```python
from build123d import *

# Parameters (mm, degrees)
SKETCH_1_R          = 1.45
EXTRUDE_1_DEPTH     = 21
EXTRUDE_2_DEPTH     = 1.3
FILLET_1_R          = 0.3
FILLET_2_R          = 0.3
SKETCH_3_R          = 1
CUT_EXTRUDE_3_DEPTH = 10
FILLET_3_R          = 2
SKETCH_4_W          = 3.3
SKETCH_4_H          = 21
EXTRUDE_4_DEPTH     = 0.6
SKETCH_7_W          = 15
SKETCH_7_H          = 13.536537926
SKETCH_7_W_2        = 10.5
SKETCH_7_H_2        = 9.5
CUT_EXTRUDE_4_DEPTH = 10
FILLET_7_R          = 3


with BuildPart() as part:
    # 草圖1 → 填料-伸長1 (new body)
    with BuildSketch(Plane(origin=(0, 0, 0), x_dir=(1, 0, 0), z_dir=(0, 1, 0))):
        Polygon((17.3, -0.9), (14.5, -0.9), (14.5, -4.2), (17.3, -4.2), (17.3, -5), (0, -5), (-2.5, -5), (-2.5, 0), (0, 0), (17.3, 0), align=None)
        with Locations(Location((0, -2.5, 0), (0, 0, 90))):
            Circle(SKETCH_1_R, mode=Mode.SUBTRACT)
    extrude(amount=EXTRUDE_1_DEPTH)

    # 草圖2 → 填料-伸長2 (add)
    with BuildSketch(Plane(origin=(14.5, 0, 0), x_dir=(0, 0, -1), z_dir=(1, 0, 0))):
        Polygon((-4.2, 5.659075235), (-0.9, 4.159075235), (-0.9, 3.5), (-4.2, 5), align=None)
        Polygon((-4.2, 2.659075235), (-0.9, 1.159075235), (-0.9, 0.5), (-4.2, 2), align=None)
        Polygon((-4.2, 17.659075235), (-0.9, 16.159075235), (-0.9, 15.5), (-4.2, 17), align=None)
        Polygon((-4.2, 20.659075235), (-0.9, 19.159075235), (-0.9, 18.5), (-4.2, 20), align=None)
    extrude(amount=EXTRUDE_2_DEPTH)

    # 圓角1
    fillet_1_edges = [part.edges().sort_by_distance(p)[0] for p in [
        (15.8, 1.909075235, 2.55),
        (15.8, 1.25, 2.55),
        (15.8, 4.25, 2.55),
        (15.8, 4.909075235, 2.55),
        (15.8, 16.25, 2.55),
        (15.8, 16.909075235, 2.55),
        (15.8, 19.25, 2.55),
        (15.8, 19.909075235, 2.55),
    ]]
    fillet(fillet_1_edges, radius=FILLET_1_R - 0.0001)  # a hair under: the kernel refuses the full size

    # 圓角2
    fillet_2_edges = [part.edges().sort_by_distance(p)[0] for p in [
        (17.3, 10.5, 0),
        (17.3, 10.5, 0.9),
        (17.3, 10.5, 4.2),
        (17.3, 10.5, 5),
    ]]
    fillet(fillet_2_edges, radius=FILLET_2_R)

    # 草圖3 → 除料-伸長3 (cut)
    with BuildSketch(Plane.XY):
        with Locations(Location((9.5, 18.5, 0), (0, 0, 180))):
            Circle(SKETCH_3_R)
    extrude(amount=CUT_EXTRUDE_3_DEPTH, mode=Mode.SUBTRACT)

    # 圓角3
    fillet_3_edges = [part.edges().sort_by_distance(p)[0] for p in [
        (-2.5, 10.5, 5),
        (-2.5, 10.5, 0),
    ]]
    fillet(fillet_3_edges, radius=FILLET_3_R)

    # 草圖4 → 填料-伸長4 (add)
    with BuildSketch(Plane(origin=(14.5, 0, 0), x_dir=(0, 0, -1), z_dir=(1, 0, 0))):
        with Locations((-2.55, 10.5)):
            Rectangle(SKETCH_4_W, SKETCH_4_H)
    extrude(amount=EXTRUDE_4_DEPTH)

    # 草圖7 → 除料-伸長4 (cut)
    with BuildSketch(Plane.XY.offset(5)):
        with Locations((4.5, -0.768268963)):
            Rectangle(SKETCH_7_W, SKETCH_7_H)
        with Locations((2.25, 18.25)):
            Rectangle(SKETCH_7_W_2, SKETCH_7_H_2)
    extrude(amount=-CUT_EXTRUDE_4_DEPTH, mode=Mode.SUBTRACT)

    # 圓角7
    fillet_7_edges = [part.edges().sort_by_distance(p)[0] for p in [
        (7.5, 21, 2.5),
    ]]
    fillet(fillet_7_edges, radius=FILLET_7_R)


solid = part.part
```
The listing builds one solid part. Answer for the finished solid, in the listing's coordinates (mm). A direction names the side the tool comes from. Give positions to 0.01 mm unless a question says otherwise; leave off trailing zeros. Order: outer loops, then holes, each group sorted by start corner. A loop starts at its lowest first (then second) coordinate and runs counter-clockwise, first axis right, second up. Notation, with made-up numbers: (72, 55.5) - (77, 55.5) arc R25 cw to (77, 67.5) - close; hole circle Ø1 at (-18.5, 29). An arc over 180 degrees is marked (long way). Answer in a Markdown table with one row per item. Add a question column.
Q1. The part is cut by section B-B (y = 8). Determine the outline of the cut face in (x, z).
Q2. The part is cut by section D-D (x = 9.5). Determine the outline of the cut face in (y, z), then the cut area to 3 significant figures.
Q3. Which of the six approach directions +Z, -Z, +X, -X, +Y, -Y give full straight-line access (tool end or side, diameter ignored) to faces 1 (the flat face through (15.1, 20, 2)), 2 (the cylindrical face through (-1.9, 9.8, 0.57)), 3 (the flat face through (15.3, 4.92, 2.57))?
Q4. The part is cut by section A-A (x = 0). Determine the outline of the cut face in (y, z).
Q5. The part is cut by section C-C (z = 2.5). Give the number of separate pieces and of enclosed holes in the cut face, then the cut area to 3 significant figures.
Q6. For a pull along Y with two mould halves and no side action, classify faces 4 (the flat face through (5, 6, 3)), 5 (the flat face through (15.3, 16.24, 2.53)), 6 (the cylindrical face through (15.7, 19.8, 2.5)), 7 (the flat face through (15.1, 1, 3)) as released by +Y, released by -Y, zero draft, split by the parting line, or undercut.
Q7. Given P1, Ø1.5, axis at y = 3.5, z = 2, coming from the -X side; P2, Ø3, axis at y = 18, z = 3, coming from the +X side; P3, Ø3, axis at y = 14.5, z = 2.5, coming from the +X side; P4, Ø0.6, axis at y = 1.5, z = 2.5, coming from the +X side, each flat-ended and moving along its own axis, determine where each tip first touches the part or whether it passes through.
Q8. Find the intervals of material crossed by line 1 along X through (y, z) = (9.5, 2.5); line 2 along Z through (x, y) = (16, 12.75); line 3 along X through (y, z) = (18.5, 2.45), in increasing order. Write a range as [from, to].
Determined:
| question | item | result |
|---|---|---|
| 1 | outline | (-2.5, 2) arc R2 ccw to (-0.5, 0) - (17, 0) arc R0.3 ccw to (17.3, 0.3) - (17.3, 0.6) arc R0.3 ccw to (17, 0.9) - (15.1, 0.9) - (15.1, 4.2) - (17, 4.2) arc R0.3 ccw to (17.3, 4.5) - (17.3, 4.7) arc R0.3 ccw to (17, 5) - (-0.5, 5) arc R2 ccw to (-2.5, 3) - close; hole circle Ø2.9 at (0, 2.5) |
| 2 | outline | (6, 0) - (17.5, 0) - (17.5, 5) - (6, 5) - close; (19.5, 0) - (20.83, 0) - (20.83, 5) - (19.5, 5) - close |
| 2 | area | 64.1 mm² |
| 3 | face 1 | +X, +Y |
| 3 | face 2 | -Z, -X, +Y, -Y |
| 3 | face 3 | +X |
| 4 | outline | (6, 0) - (13.5, 0) - (13.5, 1.05) - (6, 1.05) - close; (6, 3.95) - (13.5, 3.95) - (13.5, 5) - (6, 5) - close |
| 5 | separate pieces | 2 |
| 5 | enclosed holes | 1 |
| 5 | area | 182 mm² |
| 6 | face 4 | released by -Y |
| 6 | face 5 | undercut |
| 6 | face 6 | released by +Y |
| 6 | face 7 | zero draft |
| 7 | P1 | stops at x = 12 |
| 7 | P2 | stops at x = 17.3 |
| 7 | P3 | stops at x = 15.1 |
| 7 | P4 | stops at x = 15.8 |
| 8 | line 1 | x = [-2.5, -1.45], [1.45, 15.1] |
| 8 | line 2 | z = [0, 0.9], [4.2, 5] |
| 8 | line 3 | x = [7.54, 8.5], [10.5, 15.1] |
